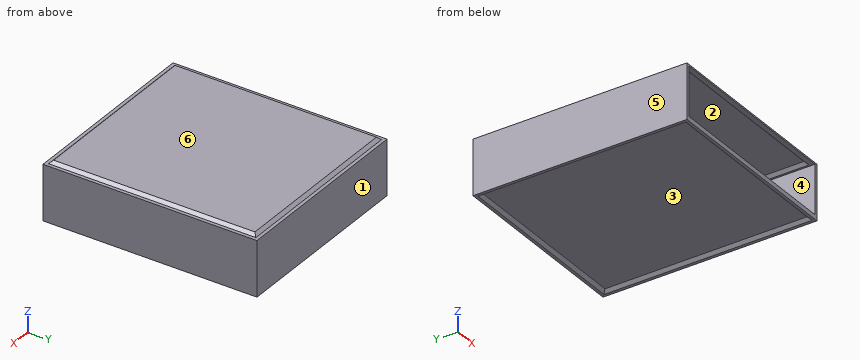
```python
from build123d import *

# Parameters (mm, degrees)
F0_W      = 129
F0_H      = 143.5
F0_W_2    = 125
F0_H_2    = 139.5
F1_DEPTH  = 3
F2_DEPTH  = 2
F3_SIZE   = 1.99999
F5_DEPTH  = 33
F6_W      = 125
F6_H      = 141.5
F6_W_2    = 124.5
F6_H_2    = 139
F6_W_3    = 122.5
F6_H_3    = 137
F7_DEPTH  = 1
F8_DEPTH  = 3
F9_SIZE   = 1.99999
F10_DEPTH = 2
F10_TAPER = 45


# Not quite as in the source:
# - a fillet or chamfer is up to 0.001 mm smaller than in the source, because OpenCascade refuses the exact size
# - a feature names something its author has since deleted; it is built from what else it names


with BuildPart() as f1:
    # F0 (on Top) → F1 (new body)
    with BuildSketch(Plane.XY):
        Rectangle(F0_W, F0_H)
        Rectangle(F0_W_2, F0_H_2, mode=Mode.SUBTRACT)
        Rectangle(F0_W_2, F0_H_2)
    extrude(amount=F1_DEPTH)

    # F0 (on Top) → F2 (cut)
    with BuildSketch(Plane.XY):
        Rectangle(F0_W_2, F0_H_2)
    extrude(amount=F2_DEPTH, mode=Mode.SUBTRACT)

    # F3 (size 2 in the source; OpenCascade refuses exactly that, so slightly less here)
    f3_edges = [f1.edges().sort_by_distance(p)[0] for p in [
        (0, -69.75, 2),
        (62.5, 0, 2),
        (0, 69.75, 2),
        (-62.5, 0, 2),
    ]]
    chamfer(f3_edges, length=F3_SIZE)

    # F4 (on face) → F5 (join)
    with BuildSketch(Plane.XY.offset(3)):
        Polygon((-64.5, 71.75), (-64.5, -71.75), (-62.5, -71.75), (-62.5, 69.75), (62.5, 69.75), (62.5, -71.75), (64.5, -71.75), (64.5, 71.75), align=None)
    extrude(amount=F5_DEPTH)

    # F6 (on face) → F7 (join)
    with BuildSketch(Plane.XY.offset(36)):
        with Locations((0, -1)):
            Rectangle(F6_W, F6_H)
        Rectangle(F6_W_2, F6_H_2, mode=Mode.SUBTRACT)
        Rectangle(F6_W_2, F6_H_2)
        Rectangle(F6_W_3, F6_H_3, mode=Mode.SUBTRACT)
        Polygon((-64.5, 71.75), (-64.5, -71.75), (-62.5, -71.75), (-62.5, 69.75), (62.5, 69.75), (62.5, -71.75), (64.5, -71.75), (64.5, 71.75), align=None)
    extrude(amount=F7_DEPTH)

    # F6 (on face) → F8 (join)
    with BuildSketch(Plane.XY.offset(36)):
        Rectangle(F6_W_2, F6_H_2)
        Rectangle(F6_W_3, F6_H_3, mode=Mode.SUBTRACT)
        Rectangle(F6_W_3, F6_H_3)
    extrude(amount=F8_DEPTH)

    # F9 (size 2 in the source; OpenCascade refuses exactly that, so slightly less here)
    f9_edges = [f1.edges().sort_by_distance(p)[0] for p in [
        (-62.25, 0, 39),
        (0, 69.5, 39),
        (0, -69.5, 39),
        (62.25, 0, 39),
    ]]
    chamfer(f9_edges, length=F9_SIZE)

    # F6 (on face) → F10 (cut)
    with BuildSketch(Plane.XY.offset(36)):
        Rectangle(F6_W_3, F6_H_3)
    extrude(amount=F10_DEPTH, taper=F10_TAPER, mode=Mode.SUBTRACT)


solid = f1.part
```
Can you work these out from the model? Positions are in its coordinate system, mm. Face numbers are marked on the shaded views. A direction names the side the tool comes from. Give positions to 0.01 mm unless a question says otherwise; leave off trailing zeros. Order: outer loops, then holes, each group sorted by start corner. A loop starts at its lowest first (then second) coordinate and runs counter-clockwise, first axis right, second up. Notation, with made-up numbers: (-0.75, 4.5) - (12.25, 4.5) arc R24 cw to (12.25, 18.5) - close; hole circle Ø8 at (19.5, -1). An arc over 180 degrees is marked (long way). Use a Markdown table: item, result. Add a question column.
Q1. If we section it at B-B on z = 10.5: Write out the boundary of the cut face in (x, y), plus the area to 3 significant figures.
Q2. Please list where these lines run through material, in increasing order: line 1 along Z through (x, y) = (39, -52); line 2 along X through (y, z) = (-26.5, 6); line 3 along Y through (x, z) = (-16, 30).
Q3. If we mould it in two halves opening along Z, with no side actions, what happens to the marked faces 4, 5 and 6? For each: released by +Z, released by -Z, zero draft, split by the parting line, or undercut.
Q4. I'm going to push flat-ended pins straight in: pin 1 (6 mm diameter, centred on x = -47.5, y = -56, fed in from -Z); pin 2 (16.5 mm diameter, centred on x = 0, z = 26.5, fed in from -Y). Where does each tip first touch, or does it pass through?
Q5. On a 3-axis mill with a long thin cutter (end or side, diameter ignored), from which of +Z, -Z, +X, -X, +Y, -Y can I reach the whole of each face in a straight line? I mean the marked faces 1, 2 and 3. Say none if no direction works.
Answers follow:
| question | item | result |
|---|---|---|
| 1 | outline | (-64.5, -71.75) - (-62.5, -71.75) - (-62.5, 69.75) - (62.5, 69.75) - (62.5, -71.75) - (64.5, -71.75) - (64.5, 71.75) - (-64.5, 71.75) - close |
| 1 | area | 824 mm^2 |
| 2 | line 1 | z = 2 to 3, 38 to 39 |
| 2 | line 2 | x = -64.5 to -62.5, 62.5 to 64.5 |
| 2 | line 3 | y = 69.75 to 71.75 |
| 3 | face 4 | undercut |
| 3 | face 5 | zero draft |
| 3 | face 6 | released by +Z |
| 4 | pin 1 | stops at z = 2 |
| 4 | pin 2 | stops at y = 69.75 |
| 5 | face 1 | +Z, -Z, +X, -X, +Y |
| 5 | face 2 | none |
| 5 | face 3 | -Z |
